```python
from build123d import *

# Parameters (mm, degrees)
BASPROSKE_W        = 11.811
BASPROSKE_H        = 28.575
TOOTHCUT_DEPTH     = 43.101792967
TEETHCUTS_COUNT    = 16
TEETHCUTS_ANGLE    = 337.5
BORSKE_R           = 0.396875
BORE_DEPTH         = 50.8000508
SKETCH1_R          = 3.175
CUT_EXTRUDE1_DEPTH = 42.540449503
SKETCH2_R          = 1.7272
CUT_EXTRUDE2_DEPTH = 42.540449503
SKETCH3_W          = 84.477604546
SKETCH3_H          = 60.621692784
CUT_EXTRUDE3_DEPTH = 7.4168


with BuildPart() as part:
    # BasProSke → Base-Revolve (revolve)
    with BuildSketch(Plane(origin=(0, 0, 0), x_dir=(1, 0, 0), z_dir=(0, 1, 0)), mode=Mode.PRIVATE) as base_revolve_sk:
        with Locations((5.9055, 14.2875)):
            Rectangle(BASPROSKE_W, BASPROSKE_H)
    revolve(base_revolve_sk.sketch.rotate(Axis((-10, 0, 0), (1, 0, 0)), 180), axis=Axis((-10, 0, 0), (1, 0, 0)))

    # TooCutSke → ToothCut (cut, through all)
    with BuildSketch(Plane(origin=(0, 0, 0), x_dir=(0, 0, -1), z_dir=(1, 0, 0))):
        with BuildLine():
            ThreePointArc((1.653773222, 21.366073035), (0, 21.42998), (-1.653773222, 21.366073035))
            ThreePointArc((-1.653773222, 21.366073035), (-2.605634946, 25.083646688), (-4.868483936, 28.182986789))
            ThreePointArc((-4.868483936, 28.182986789), (0, 28.6004), (4.868483936, 28.182986789))
            ThreePointArc((4.868483936, 28.182986789), (2.605634946, 25.083646688), (1.653773222, 21.366073035))
        make_face()
    toothcut = extrude(amount=TOOTHCUT_DEPTH, mode=Mode.SUBTRACT)

    # TeethCuts: ToothCut ×16 about axis
    teethcuts_axis = Axis((-10, 0, 0), (1, 0, 0))
    for i in range(1, TEETHCUTS_COUNT):
        add(toothcut.rotate(teethcuts_axis, i * TEETHCUTS_ANGLE / (TEETHCUTS_COUNT - 1)), mode=Mode.SUBTRACT)

    # BorSke → Bore (cut, symmetric)
    with BuildSketch(Plane(origin=(0, 0, 0), x_dir=(0, 0, -1), z_dir=(1, 0, 0))):
        with Locations(Location((0, 0, 0), (0, 0, 180))):
            Circle(BORSKE_R)
    extrude(amount=BORE_DEPTH, both=True, mode=Mode.SUBTRACT)

    # Sketch1 → Cut-Extrude1 (cut, through all)
    with BuildSketch(Plane(origin=(11.811, 0, 0), x_dir=(0, 0, -1), z_dir=(1, 0, 0))):
        Circle(SKETCH1_R)
    extrude(amount=-CUT_EXTRUDE1_DEPTH, mode=Mode.SUBTRACT)

    # Sketch2 → Cut-Extrude2 (cut, through all)
    with BuildSketch(Plane(origin=(11.811, 0, 0), x_dir=(0, 0, -1), z_dir=(1, 0, 0))):
        with Locations((0, 15.24)):
            Circle(SKETCH2_R)
        with Locations((14.494101308, 4.709418994)):
            Circle(SKETCH2_R)
        with Locations((8.957847245, -12.329418994)):
            Circle(SKETCH2_R)
        with Locations((-8.957847245, -12.329418994)):
            Circle(SKETCH2_R)
        with Locations((-14.494101308, 4.709418994)):
            Circle(SKETCH2_R)
    extrude(amount=-CUT_EXTRUDE2_DEPTH, mode=Mode.SUBTRACT)

    # Sketch3 → Cut-Extrude3 (cut)
    with BuildSketch(Plane.ZY):
        with Locations((1.281804372, -1.088129041)):
            Rectangle(SKETCH3_W, SKETCH3_H)
    extrude(amount=-CUT_EXTRUDE3_DEPTH, mode=Mode.SUBTRACT)


solid = part.part
```
The model under review builds one solid part; all positions refer to its coordinate system, in mm. A direction names the side the tool comes from. Give positions to 0.01 mm unless a question says otherwise; leave off trailing zeros. Write each loop counter-clockwise with the first axis right and the second up, starting at its lowest first coordinate (ties: lowest second). Pieces come first, ordered by that corner, then holes. Notation, with made-up numbers: (-8.5, 77.25) -> (44.5, 77.25) arc R31 cw to (44.5, 109.25) -> close; hole circle Ø3 at (-18, 40.5). An arc over 180 degrees is marked (long way). Put each result on its own line as item: value.
(1) Tool access review of faces 4 (the cylindrical face through (9.583, -15.17, -15.137)), 5 (the cylindrical face through (9.583, 11.955, -22.13)), 6 (the cylindrical face through (9.583, 2.622, 25.118)), 7 (the cylindrical face through (9.583, 25.02, 2.576)): name each direction out of +Z, -Z, +X, -X, +Y, -Y from which nothing blocks a thin tool from reaching the whole face with its end or side.
Results are:
face 4: +X, -X
face 5: -Z, +X, -X
face 6: +Z, +X, -X
face 7: +X, -X, +Y
(2) We need section A-A, the plane z = 0. Give the boundary of the cut face in (x, y) (3 decimals).
Results are:
outline: (7.417, -21.43) -> (11.811, -21.43) -> (11.811, -3.175) -> (7.417, -3.175) -> close; (7.417, 3.175) -> (11.811, 3.175) -> (11.811, 13.513) -> (7.417, 13.513) -> close; (7.417, 16.967) -> (11.811, 16.967) -> (11.811, 21.43) -> (7.417, 21.43) -> close
(3) For pin 1 Ø4 at (y, z) = (-12.33, 8.96) entering from -X; pin 2 Ø4 at (y, z) = (0, 0) entering from +X; pin 3 Ø2 at (x, z) = (11, 9.5) entering from +Y; pin 4 Ø1 at (x, z) = (10, -17.5) entering from +Y, all flat-tipped, find the tip position at first contact; note any pin that passes through.
Results are:
pin 1: x = 7.42
pin 2: through
pin 3: y = 20.46
pin 4: y = 15.17
(4) We need section C-C, the plane y = -11.5. Give the boundary of the cut face in (x, z).
Results are:
outline: (7.42, -21.68) -> (11.81, -21.68) -> (11.81, -10.47) -> (7.42, -10.47) -> close; (7.42, -7.44) -> (11.81, -7.44) -> (11.81, 7.44) -> (7.42, 7.44) -> close; (7.42, 10.47) -> (11.81, 10.47) -> (11.81, 21.68) -> (7.42, 21.68) -> close
(5) The part is to be moulded in two halves that separate along Y. For faces 1 (the cylindrical face through (9.58, -12.03, -22.2)), 2 (the cylindrical face through (9.645, 23.753, -15.884)), 3 (the cylindrical face through (9.645, -15.884, -23.753)), say which applies: pulls with the +Y half, pulls with the -Y half, needs draft (parallel to the pull), parting line crosses it, or undercut.
Results are:
face 1: undercut
face 2: pulls with the +Y half
face 3: pulls with the -Y half
(6) We need section B-B, the plane y = 0. Give the boundary of the cut face in (x, z) (3 decimals).
Results are:
outline: (7.417, -21.43) -> (11.811, -21.43) -> (11.811, -3.175) -> (7.417, -3.175) -> close; (7.417, 3.175) -> (11.811, 3.175) -> (11.811, 21.43) -> (7.417, 21.43) -> close
(7) We need section D-D, the plane x = 10.8. State how many separate pieces and enclosed holes the cut face has, and give its area (3 significant figures).
Results are:
separate pieces: 1
enclosed holes: 6
area: 1,860 mm²
(8) To check wall thickness, follow probe 1 along Y at (x, z) = (11.35, 23); probe 2 along Y at (x, z) = (9.65, 1); probe 3 along Z at (x, y) = (11.65, -21.5). State the ranges of each line that lie inside material, in increasing order. Write a range as from..to.
Results are:
probe 1: -16.49..-13.04, -7.18..-1.89, 1.89..7.18, 13.04..16.49
probe 2: -21.41..-3.01, 3.01..13.83, 16.65..21.41
probe 3: -16.38..-11.33, -6.97..-1.66, 1.66..6.97, 11.33..16.38
